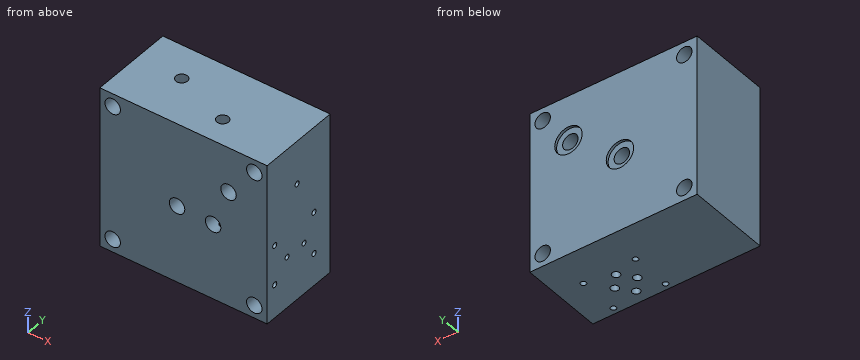
from build123d import *

# Parameters (mm, degrees)
SKETCH_2_W                 = 130
SKETCH_2_H                 = 125
SKETCH_2_R                 = 6
EXTRUDE_1_DEPTH            = 65
HOLE_WIZARD_M5_3_D         = 4.2
HOLE_WIZARD_M5_3_DEPTH     = 12
HOLE_WIZARD_M5_3_TIP       = 1.2618073
HOLE_WIZARD_4_0_4_9_D      = 4
HOLE_WIZARD_4_0_4_9_DEPTH  = 32.5
HOLE_WIZARD_4_0_4_9_TIP    = 1.201721238
HOLE_WIZARD_6_0_6_1_D      = 6
HOLE_WIZARD_6_0_6_1_DEPTH  = 42
HOLE_WIZARD_6_0_6_1_TIP    = 1.802581857
HOLE_WIZARD_4_0_4_11_D     = 4
HOLE_WIZARD_4_0_4_11_DEPTH = 85
HOLE_WIZARD_4_0_4_11_TIP   = 1.201721238
M10X1_0_1_D                = 9
M10X1_0_1_DEPTH            = 13
M10X1_0_1_TIP              = 2.703872786
HOLE_WIZARD_M5_5_D         = 4.2
HOLE_WIZARD_M5_5_DEPTH     = 10
HOLE_WIZARD_M5_5_TIP       = 1.2618073
HOLE_WIZARD_6_0_6_2_D      = 6
HOLE_WIZARD_6_0_6_2_DEPTH  = 60
HOLE_WIZARD_6_0_6_2_TIP    = 1.802581857
HOLE_WIZARD_6_0_6_3_D      = 6
HOLE_WIZARD_6_0_6_3_DEPTH  = 90
HOLE_WIZARD_6_0_6_3_TIP    = 1.802581857
HOLE_WIZARD_M5_8_D         = 4.2
HOLE_WIZARD_M5_8_DEPTH     = 41.31
HOLE_WIZARD_M5_8_TIP       = 1.2618073
HOLE_WIZARD_6_0_6_4_D      = 6
M10X1_0_2_D                = 9
M10X1_0_2_DEPTH            = 13
M10X1_0_2_TIP              = 2.703872786
SKETCH_73_R                = 10.65
CUT_EXTRUDE_1_DEPTH        = 1.97
SKETCH_74_R                = 6
CUT_EXTRUDE_2_DEPTH        = 64.03
SKETCH_75_R                = 10.65
CUT_EXTRUDE_3_DEPTH        = 1.97
SKETCH_76_R                = 6
CUT_EXTRUDE_4_DEPTH        = 64.03
SKETCH_82_R                = 2
CUT_EXTRUDE_6_DEPTH        = 97
SKETCH_83_R                = 6
CUT_EXTRUDE_7_DEPTH        = 13


with BuildPart() as part:
    # 草图2 → 凸台-拉伸1 (new body)
    with BuildSketch(Plane(origin=(0, 0, 0), x_dir=(1, 0, 0), z_dir=(0, 1, 0))):
        Rectangle(SKETCH_2_W, SKETCH_2_H)
        with Locations((-55, 52.5)):
            Circle(SKETCH_2_R, mode=Mode.SUBTRACT)
        with Locations((55, 52.5)):
            Circle(SKETCH_2_R, mode=Mode.SUBTRACT)
        with Locations((55, -52.5)):
            Circle(SKETCH_2_R, mode=Mode.SUBTRACT)
        with Locations((-55, -52.5)):
            Circle(SKETCH_2_R, mode=Mode.SUBTRACT)
    extrude(amount=EXTRUDE_1_DEPTH)

    # M5 螺纹孔3
    with Locations(Plane(origin=(65, 48.3, -4.65), x_dir=(0, 0, 1), z_dir=(1, 0, 0))):
        with Locations((0, 0), (-32.5, 0), (-31.75, 40.5), (-0.75, 40.5)):
            Hole(HOLE_WIZARD_M5_3_D / 2, depth=HOLE_WIZARD_M5_3_DEPTH)
            with Locations((0, 0, -(HOLE_WIZARD_M5_3_DEPTH + HOLE_WIZARD_M5_3_TIP / 2))):  # 118° drill point
                Cone(0, HOLE_WIZARD_M5_3_D / 2, HOLE_WIZARD_M5_3_TIP, mode=Mode.SUBTRACT)

    # Ø4.0 (4) 直径孔9
    with Locations(Plane(origin=(65, 20.5, -22.49541266), x_dir=(0, 0, 1), z_dir=(1, 0, 0))):
        with Locations((0, 0)):
            Hole(HOLE_WIZARD_4_0_4_9_D / 2, depth=HOLE_WIZARD_4_0_4_9_DEPTH)
            with Locations((0, 0, -(HOLE_WIZARD_4_0_4_9_DEPTH + HOLE_WIZARD_4_0_4_9_TIP / 2))):  # 118° drill point
                Cone(0, HOLE_WIZARD_4_0_4_9_D / 2, HOLE_WIZARD_4_0_4_9_TIP, mode=Mode.SUBTRACT)

    # Ø6.0 (6) 直径孔1
    with Locations(Plane(origin=(32.5, 20.5, -62.5), x_dir=(-1, 0, 0), z_dir=(0, 0, -1))):
        with Locations((0, 0)):
            Hole(HOLE_WIZARD_6_0_6_1_D / 2, depth=HOLE_WIZARD_6_0_6_1_DEPTH)
            with Locations((0, 0, -(HOLE_WIZARD_6_0_6_1_DEPTH + HOLE_WIZARD_6_0_6_1_TIP / 2))):  # 118° drill point
                Cone(0, HOLE_WIZARD_6_0_6_1_D / 2, HOLE_WIZARD_6_0_6_1_TIP, mode=Mode.SUBTRACT)

    # Ø4.0 (4) 直径孔11
    with Locations(Plane(origin=(-30, 38, 62.5), x_dir=(1, 0, 0), z_dir=(0, 0, 1))):
        with Locations((0, 0)):
            Hole(HOLE_WIZARD_4_0_4_11_D / 2, depth=HOLE_WIZARD_4_0_4_11_DEPTH)
            with Locations((0, 0, -(HOLE_WIZARD_4_0_4_11_DEPTH + HOLE_WIZARD_4_0_4_11_TIP / 2))):  # 118° drill point
                Cone(0, HOLE_WIZARD_4_0_4_11_D / 2, HOLE_WIZARD_4_0_4_11_TIP, mode=Mode.SUBTRACT)

    # M10x1.0 螺纹孔1
    with Locations(Plane(origin=(-30, 38, 62.5), x_dir=(1, 0, 0), z_dir=(0, 0, 1))):
        with Locations((0, 0)):
            Hole(M10X1_0_1_D / 2, depth=M10X1_0_1_DEPTH)
            with Locations((0, 0, -(M10X1_0_1_DEPTH + M10X1_0_1_TIP / 2))):  # 118° drill point
                Cone(0, M10X1_0_1_D / 2, M10X1_0_1_TIP, mode=Mode.SUBTRACT)

    # M5 螺纹孔5
    with Locations(Plane(origin=(4.7, 36, -62.5), x_dir=(-1, 0, 0), z_dir=(0, 0, -1))):
        with Locations((0, 0), (-40.5, 0), (-40.5, -31), (0, -31)):
            Hole(HOLE_WIZARD_M5_5_D / 2, depth=HOLE_WIZARD_M5_5_DEPTH)
            with Locations((0, 0, -(HOLE_WIZARD_M5_5_DEPTH + HOLE_WIZARD_M5_5_TIP / 2))):  # 118° drill point
                Cone(0, HOLE_WIZARD_M5_5_D / 2, HOLE_WIZARD_M5_5_TIP, mode=Mode.SUBTRACT)

    # Ø6.0 (6) 直径孔2
    with Locations(Plane(origin=(23.7, 10.1, -62.5), x_dir=(-1, 0, 0), z_dir=(0, 0, -1))):
        with Locations((0, 0)):
            Hole(HOLE_WIZARD_6_0_6_2_D / 2, depth=HOLE_WIZARD_6_0_6_2_DEPTH)
            with Locations((0, 0, -(HOLE_WIZARD_6_0_6_2_DEPTH + HOLE_WIZARD_6_0_6_2_TIP / 2))):  # 118° drill point
                Cone(0, HOLE_WIZARD_6_0_6_2_D / 2, HOLE_WIZARD_6_0_6_2_TIP, mode=Mode.SUBTRACT)

    # Ø6.0 (6) 直径孔3
    with Locations(Plane(origin=(23.7, 30.9, -62.5), x_dir=(-1, 0, 0), z_dir=(0, 0, -1))):
        with Locations((0, 0)):
            Hole(HOLE_WIZARD_6_0_6_3_D / 2, depth=HOLE_WIZARD_6_0_6_3_DEPTH)
            with Locations((0, 0, -(HOLE_WIZARD_6_0_6_3_DEPTH + HOLE_WIZARD_6_0_6_3_TIP / 2))):  # 118° drill point
                Cone(0, HOLE_WIZARD_6_0_6_3_D / 2, HOLE_WIZARD_6_0_6_3_TIP, mode=Mode.SUBTRACT)

    # M5 螺纹孔8
    with Locations(Plane(origin=(65, 30.9, 28.70458734), x_dir=(0, 0, 1), z_dir=(1, 0, 0))):
        with Locations((0, 0)):
            Hole(HOLE_WIZARD_M5_8_D / 2, depth=HOLE_WIZARD_M5_8_DEPTH)
            with Locations((0, 0, -(HOLE_WIZARD_M5_8_DEPTH + HOLE_WIZARD_M5_8_TIP / 2))):  # 118° drill point
                Cone(0, HOLE_WIZARD_M5_8_D / 2, HOLE_WIZARD_M5_8_TIP, mode=Mode.SUBTRACT)

    # Ø6.0 (6) 直径孔4 (through all)
    with Locations(Plane(origin=(15, 20.5, -62.5), x_dir=(-1, 0, 0), z_dir=(0, 0, -1))):
        with Locations((0, 0)):
            Hole(HOLE_WIZARD_6_0_6_4_D / 2)

    # M10x1.0 螺纹孔2
    with Locations(Plane(origin=(15, 20.5, 62.5), x_dir=(1, 0, 0), z_dir=(0, 0, 1))):
        with Locations((0, 0)):
            Hole(M10X1_0_2_D / 2, depth=M10X1_0_2_DEPTH)
            with Locations((0, 0, -(M10X1_0_2_DEPTH + M10X1_0_2_TIP / 2))):  # 118° drill point
                Cone(0, M10X1_0_2_D / 2, M10X1_0_2_TIP, mode=Mode.SUBTRACT)

    # 草图73 → 切除-拉伸1 (cut)
    with BuildSketch(Plane(origin=(0, 65, 0), x_dir=(1, 0, 0), z_dir=(0, 1, 0))):
        with Locations((-5, 2.5)):
            Circle(SKETCH_73_R)
    extrude(amount=-CUT_EXTRUDE_1_DEPTH, mode=Mode.SUBTRACT)

    # 草图74 → 切除-拉伸2 (cut, through all)
    with BuildSketch(Plane(origin=(0, 63.03, 0), x_dir=(1, 0, 0), z_dir=(0, 1, 0))):
        with Locations((-5, 2.5)):
            Circle(SKETCH_74_R)
    extrude(amount=-CUT_EXTRUDE_2_DEPTH, mode=Mode.SUBTRACT)

    # 草图75 → 切除-拉伸3 (cut)
    with BuildSketch(Plane(origin=(0, 65, 0), x_dir=(1, 0, 0), z_dir=(0, 1, 0))):
        with Locations((35, -27.5)):
            Circle(SKETCH_75_R)
    extrude(amount=-CUT_EXTRUDE_3_DEPTH, mode=Mode.SUBTRACT)

    # 草图76 → 切除-拉伸4 (cut, through all)
    with BuildSketch(Plane(origin=(0, 63.03, 0), x_dir=(1, 0, 0), z_dir=(0, 1, 0))):
        with Locations((35, -27.5)):
            Circle(SKETCH_76_R)
    extrude(amount=-CUT_EXTRUDE_4_DEPTH, mode=Mode.SUBTRACT)

    # 草图82 → 切除-拉伸6 (cut)
    with BuildSketch(Plane(origin=(65, 0, 0), x_dir=(0, 0, -1), z_dir=(1, 0, 0))):
        with Locations((22.5, 38)):
            Circle(SKETCH_82_R)
    extrude(amount=-CUT_EXTRUDE_6_DEPTH, mode=Mode.SUBTRACT)

    # 草图83 → 切除-拉伸7 (cut)
    with BuildSketch(Plane(origin=(0, 0, 0), x_dir=(-1, 0, 0), z_dir=(0, -1, 0))):
        with Locations((-23, 3.7)):
            Circle(SKETCH_83_R)
    extrude(amount=-CUT_EXTRUDE_7_DEPTH, mode=Mode.SUBTRACT)


solid = part.part
Here's how the part is built. I have some questions about the finished solid (model axes, mm). Coordinates: 2 decimals unless noted, no trailing zeros. Write each loop counter-clockwise with the first axis right and the second up, starting at its lowest first coordinate (ties: lowest second). Pieces come first, ordered by that corner, then holes.
1) If we section it at B-B (y = 52): List the corners of the cut face in (x, z) for me.
Filled in:
outline: (-65, -62.5) - (65, -62.5) - (65, 62.5) - (-65, 62.5) - close; hole circle Ø12 at (-55, -52.5); hole circle Ø12 at (-55, 52.5); hole circle Ø12 at (-5, -2.5); hole circle Ø12 at (35, 27.5); hole circle Ø12 at (55, -52.5); hole circle Ø12 at (55, 52.5)
2) If we section it at C-C (x = 15): List the corners of the cut face in (y, z) for me.
Filled in:
outline: (0, -62.5) - (17.5, -62.5) - (17.5, 48.6) - (16, 49.5) - (16, 62.5) - (0, 62.5) - close; (23.5, -62.5) - (65, -62.5) - (65, 62.5) - (25, 62.5) - (25, 49.5) - (23.5, 48.6) - close; hole circle Ø4 at (38, -22.5)
3) If we section it at A-A (x = -5): List the corners of the cut face in (y, z) for me.
Filled in:
outline: (0, -62.5) - (65, -62.5) - (65, -13.15) - (63.03, -13.15) - (63.03, -8.5) - (0, -8.5) - close; (0, 3.5) - (63.03, 3.5) - (63.03, 8.15) - (65, 8.15) - (65, 62.5) - (0, 62.5) - close; hole circle Ø4 at (38, -22.5)
4) If I drill on line 1 (X direction, y = 26, z = -52.5); line 2 (X direction, y = 30.9, z = -4); line 3 (Z direction, x = 55, y = 19), over which ranges is the centre line in solid material (lowest first)?
Filled in:
line 1: x = -65 to -61, -49 to 49, 61 to 65
line 2: x = -65 to -10.81, 0.81 to 20.7, 26.7 to 65
line 3: z = -62.5 to -58.5, -46.5 to -23.82, -21.17 to 46.5, 58.5 to 62.5
5) I'm going to push flat-ended pins straight in: pin 1 (19 mm diameter, centred on x = -5, z = -2.5, fed in from +Y); pin 2 (4 mm diameter, centred on x = 23.5, z = -7, fed in from -Y); pin 3 (2.5 mm diameter, centred on y = 20.5, z = -22.5, fed in from +X). Where does each tip first touch, or does it pass through?
Filled in:
pin 1: stops at y = 63.03
pin 2: stops at y = 13
pin 3: stops at x = 29.77
